Source: CAD feature listing. Evaluate the final solid. Frame: model axes, mm. Round coordinates to 2 decimals unless told otherwise and drop trailing zeros. Loops run counter-clockwise (first coordinate to the right, second up) from the corner with the lowest first, then second, coordinate; pieces in that order, holes last. Notation, with made-up numbers: M -15,-25.75 L 6,-25.75 A17 ccw 6,-1.75 Z; hole C -13.5,26 d4. An arc over 180 degrees is marked long. Answer as a JSON object with one key per item and string values.
from build123d import *

# Parameters (mm, degrees)
RESSALTO_EXTRUS_O1_DEPTH = 40
ESBO_O2_R                = 5
CORTE_EXTRUS_O1_DEPTH    = 51
ESBO_O3_R                = 2.5
RESSALTO_EXTRUS_O2_DEPTH = 5
ESBO_O4_W                = 80.158201918
ESBO_O4_H                = 76.08775654
CORTE_EXTRUS_O2_DEPTH    = 50


with BuildPart() as part:
    # Esboço1 → Ressalto-extrusão1 (new body)
    with BuildSketch(Plane.XY):
        Polygon((0, 0), (0, 50), (10, 50), (10, 10), (40, 10), (40, 50), (50, 50), (50, 0), align=None)
    extrude(amount=RESSALTO_EXTRUS_O1_DEPTH)

    # Esboço2 → Corte-extrusão1 (cut, through all)
    with BuildSketch(Plane.ZY):
        with Locations((20, 33.697961809)):
            Circle(ESBO_O2_R)
    extrude(amount=-CORTE_EXTRUS_O1_DEPTH, mode=Mode.SUBTRACT)

    # Esboço3 → Ressalto-extrusão2 (add)
    with BuildSketch(Plane.ZY):
        with BuildLine():
            Line((8.284737573, 33.697961809), (8.284737573, 133.697961809))
            ThreePointArc((8.284737573, 133.697961809), (20, 145.413224236), (31.715262427, 133.697961809))
            Line((31.715262427, 133.697961809), (31.715262427, 33.697961809))
            ThreePointArc((31.715262427, 33.697961809), (20, 21.982699383), (8.284737573, 33.697961809))
        make_face()
        with Locations((15, 135.413224236)):
            Circle(ESBO_O3_R, mode=Mode.SUBTRACT)
        with Locations((25, 135.413224236)):
            Circle(ESBO_O3_R, mode=Mode.SUBTRACT)
        with Locations((25, 125.413224236)):
            Circle(ESBO_O3_R, mode=Mode.SUBTRACT)
        with Locations((15, 125.413224236)):
            Circle(ESBO_O3_R, mode=Mode.SUBTRACT)
        with Locations((25, 31.982699383)):
            Circle(ESBO_O3_R, mode=Mode.SUBTRACT)
        with Locations((25, 41.982699383)):
            Circle(ESBO_O3_R, mode=Mode.SUBTRACT)
        with Locations((15, 41.982699383)):
            Circle(ESBO_O3_R, mode=Mode.SUBTRACT)
        with Locations((15, 31.982699383)):
            Circle(ESBO_O3_R, mode=Mode.SUBTRACT)
    extrude(amount=RESSALTO_EXTRUS_O2_DEPTH)

    # Esboço4 → Corte-extrusão2 (cut)
    with BuildSketch(Plane(origin=(50, 0, 0), x_dir=(0, 0, -1), z_dir=(1, 0, 0))):
        with Locations((-9.829245476, 29.588761993)):
            Rectangle(ESBO_O4_W, ESBO_O4_H)
    extrude(amount=-CORTE_EXTRUS_O2_DEPTH, mode=Mode.SUBTRACT)


solid = part.part
Item 1: Section B-B on x = -1.9. Give the number of separate pieces and of enclosed holes in the cut face, then the cut area to 3 significant figures.
Answer sheet:
{"separate pieces": "1", "enclosed holes": "8", "area": "2,620 mm²"}
Item 2: Section A-A on y = 40.5. Return the cut outline in (x, z).
Answer sheet:
{"outline": "M -5,8.28 L 0,8.28 L 0,12.99 L -5,12.99 Z; M -5,17.01 L 0,17.01 L 0,22.99 L -5,22.99 Z; M -5,27.01 L 0,27.01 L 0,31.72 L -5,31.72 Z"}
Item 3: Section D-D on z = 29. Return the cut outline in (x, y).
Answer sheet:
{"outline": "M -5,26.2 L 0,26.2 L 0,141.2 L -5,141.2 Z"}
Item 4: Line query: probe 1 along Z at (x, y) = (-3.3, 125); probe 2 along Y at (x, z) = (-0.4, 12.75); probe 3 along Y at (x, z) = (-1.55, 23.5). Output: solid intervals per line, ascending. Write a range as from..to.
Answer sheet:
{"probe 1": "z = 8.28..12.53, 17.47..22.53, 27.47..31.72", "probe 2": "y = 24.5..30.89, 33.07..40.89, 43.07..124.32, 126.5..134.32, 136.5..142.9", "probe 3": "y = 22.52..29.98, 33.98..39.98, 43.98..123.41, 127.41..133.41, 137.41..144.88"}
Item 5: Contact query for flat-ended pins moving along their axis: pin 1 Ø6 at (y, z) = (41.98, 25) entering from +X; pin 2 Ø4.5 at (y, z) = (135.41, 25) entering from +X; pin 3 Ø1.5 at (x, z) = (-2.5, 27) entering from +Y. Output: stop coordinate, or through.
Answer sheet:
{"pin 1": "stops at x = 0", "pin 2": "passes through", "pin 3": "stops at y = 143.61"}
Item 6: Pull-direction query (Z, two-part tool) for faces 1 (the cylindrical face through (-2.465, 21.986, 20.258)), 2 (the cylindrical face through (-2.46, 29.54, 14.46)), 3 (the flat face through (-2, 84, 31.715)), 4 (the cylindrical face through (-2.465, 122.973, 24.458)); classes: pulls with the +Z half, pulls with the -Z half, needs draft (parallel to the pull), parting line crosses it, or undercut.
Answer sheet:
{"face 1": "parting line crosses it", "face 2": "undercut", "face 3": "pulls with the +Z half", "face 4": "undercut"}
Item 7: Section C-C on z = 15. Return the cut outline in (x, y).
Answer sheet:
{"outline": "M -5,23.1 L 0,23.1 L 0,29.48 L -5,29.48 Z; M -5,34.48 L 0,34.48 L 0,39.48 L -5,39.48 Z; M -5,44.48 L 0,44.48 L 0,122.91 L -5,122.91 Z; M -5,127.91 L 0,127.91 L 0,132.91 L -5,132.91 Z; M -5,137.91 L 0,137.91 L 0,144.29 L -5,144.29 Z"}
